from build123d import *

# Parameters (mm, degrees)
SKETCH2_W             = 50
SKETCH2_H             = 50
SKETCH2_W_2           = 36.5
SKETCH2_H_2           = 36.5
BOSS_EXTRUDE2_DEPTH   = 5
SKETCH1_W             = 50
SKETCH1_H             = 50
SKETCH1_W_2           = 40.5
SKETCH1_H_2           = 40.5
BOSS_EXTRUDE4_DEPTH   = 40
BOSS_EXTRUDE5_START   = -25
BOSS_EXTRUDE5_DEPTH   = 50
BOSS_EXTRUDE5_2_DEPTH = 4.75
BOSS_EXTRUDE5_START_2 = 20.25
BOSS_EXTRUDE5_3_DEPTH = 4.75
SKETCH7_W             = 50.771330761
SKETCH7_H             = 17
BOSS_EXTRUDE6_DEPTH   = 5
SKETCH8_R             = 1.6
CUT_EXTRUDE1_DEPTH    = 13.5


# Read off the part's stored shape, not the designer's step: Boss-Extrude5
with BuildPart() as part:
    # Sketch2 → Boss-Extrude2 (new body)
    with BuildSketch(Plane(origin=(0, 0, 0), x_dir=(1, 0, 0), z_dir=(0, 1, 0))):
        Rectangle(SKETCH2_W, SKETCH2_H)
        Rectangle(SKETCH2_W_2, SKETCH2_H_2, mode=Mode.SUBTRACT)
    extrude(amount=BOSS_EXTRUDE2_DEPTH)

    # Sketch1 → Boss-Extrude4 (add)
    with BuildSketch(Plane(origin=(0, 0, 0), x_dir=(1, 0, 0), z_dir=(0, 1, 0))):
        Rectangle(SKETCH1_W, SKETCH1_H)
        Rectangle(SKETCH1_W_2, SKETCH1_H_2, mode=Mode.SUBTRACT)
    extrude(amount=BOSS_EXTRUDE4_DEPTH)

    # Boss-Extrude5 outline → Boss-Extrude5 (add)
    with BuildSketch(Plane.XY.offset(BOSS_EXTRUDE5_START)):
        Polygon((25, 40), (25, 48.81635), (20.25, 47.97879675), (20.25, 40), align=None)
        Polygon((-20.25, 40), (-20.25, 40.83755325), (-25, 40), align=None)
    extrude(amount=BOSS_EXTRUDE5_DEPTH)

    # Boss-Extrude5 2 outline → Boss-Extrude5 2 (add)
    with BuildSketch(Plane.XY.offset(BOSS_EXTRUDE5_START)):
        Polygon((20.25, 40), (20.25, 47.97879675), (-20.25, 40.83755325), (-20.25, 40), align=None)
    extrude(amount=BOSS_EXTRUDE5_2_DEPTH)

    # Boss-Extrude5 3 outline → Boss-Extrude5 3 (add)
    with BuildSketch(Plane.XY.offset(BOSS_EXTRUDE5_START_2)):
        Polygon((20.25, 40), (20.25, 47.97879675), (-20.25, 40.83755325), (-20.25, 40), align=None)
    extrude(amount=BOSS_EXTRUDE5_3_DEPTH)

    # Sketch7 → Boss-Extrude6 (add)
    with BuildSketch(Plane(origin=(-7.59424597, 43.069104391, 0), x_dir=(0.984807749763281, 0.17364819609251012, 0), z_dir=(-0.17364819609251012, 0.984807749763281, 0))):
        with Locations((7.71139948, 33.5)):
            Rectangle(SKETCH7_W, SKETCH7_H)
        with Locations((7.71139948, -33.5)):
            Rectangle(SKETCH7_W, SKETCH7_H)
    extrude(amount=-BOSS_EXTRUDE6_DEPTH)

    # Sketch8 → Cut-Extrude1 (cut)
    with BuildSketch(Plane(origin=(-7.59424597, 43.069104391, 0), x_dir=(0.984807749763281, 0.17364819609251012, 0), z_dir=(-0.17364819609251012, 0.984807749763281, 0))):
        with Locations(Location((-14.1742659, -33.5, 0), (0, 0, 180))):
            Circle(SKETCH8_R)
        with Locations((29.597064861, -33.5)):
            Circle(SKETCH8_R)
        with Locations(Location((29.597064861, 33.5, 0), (0, 0, 180))):
            Circle(SKETCH8_R)
        with Locations(Location((-14.1742659, 33.5, 0), (0, 0, 180))):
            Circle(SKETCH8_R)
    extrude(amount=-CUT_EXTRUDE1_DEPTH, mode=Mode.SUBTRACT)


solid = part.part
Geometry check sheet. Reference: the model listing, model coordinates, mm. A direction names the side the tool comes from. Round coordinates to 2 decimals unless told otherwise and drop trailing zeros. Write each loop counter-clockwise with the first axis right and the second up, starting at its lowest first coordinate (ties: lowest second). Pieces come first, ordered by that corner, then holes.
Item 1: Section check D-D (y = 3.5). Record the boundary of the cut face in (x, z), plus the area to 3 significant figures.
Determined:
outline: (-25, -25) - (25, -25) - (25, 25) - (-25, 25) - close; hole (-18.25, -18.25) - (18.25, -18.25) - (18.25, 18.25) - (-18.25, 18.25) - close
area: 1,170 mm2
Item 2: Go/stop test with flat-tipped pins: pin 1 Ø5.5 at (y, z) = (3, -1) entering from +X; pin 2 Ø22 at (x, y) = (12.5, 12) entering from -Z; pin 3 Ø1.5 at (x, y) = (16, 36.5) entering from +Z. Record where each tip stops, or that it passes through.
Determined:
pin 1: stops at x = 25
pin 2: stops at z = -25
pin 3: stops at z = 25
Item 3: Material ranges on line 1 along X through (y, z) = (32.5, 20); line 2 along Z through (x, y) = (10.5, 46), recorded low to high.
Determined:
line 1: x = -25 to -20.25, 20.25 to 25
line 2: z = -42 to -20.25, 20.25 to 42
Item 4: Section check A-A (y = 16). Record the boundary of the cut face in (x, z).
Determined:
outline: (-25, -25) - (25, -25) - (25, 25) - (-25, 25) - close; hole (-20.25, -20.25) - (20.25, -20.25) - (20.25, 20.25) - (-20.25, 20.25) - close
Item 5: Section check C-C (x = -10.5). Record the boundary of the cut face in (y, z), plus the area to 3 significant figures.
Determined:
outline: (0, -25) - (37.48, -25) - (37.48, -42) - (42.56, -42) - (42.56, -20.25) - (5, -20.25) - (5, -18.25) - (0, -18.25) - close; (0, 18.25) - (5, 18.25) - (5, 20.25) - (42.56, 20.25) - (42.56, 42) - (37.48, 42) - (37.48, 25) - (0, 25) - close
area: 597 mm2
Item 6: Access from +Z, -Z, +X, -X, +Y, -Y to the whole of each face (thin tool, end or side, straight path). Record for faces 1 (the face through (25.428, 46.389, 33.619)), 2 (the face through (0, 2, 18.25)), 3 (the face through (-20.25, 23, 0)).
Determined:
face 1: +Z, -Z, +X, +Y
face 2: +Y, -Y
face 3: +Y
Item 7: Mould release check, pull along X, two halves, no side actions. Record for faces 4 (the face through (0, 22, -25)), 5 (the face through (22.71, 45.91, 34.92)), 6 (the face through (0.518, 39.422, 33.381)), 7 (the face through (-22.57, 40.43, -0.59)): +X half, -X half, draft (parallel to the pull), parting line (faces both ways), or undercut.
Determined:
face 4: draft
face 5: undercut
face 6: +X half
face 7: -X half
Item 8: Section check B-B (z = -11). Record the boundary of the cut face in (x, y), plus the area to 3 significant figures.
Determined:
outline: (-25, 0) - (-18.25, 0) - (-18.25, 5) - (-20.25, 5) - (-20.25, 40.84) - (-25, 40) - close; (18.25, 0) - (25, 0) - (25, 48.82) - (20.25, 47.98) - (20.25, 5) - (18.25, 5) - close
area: 442 mm2
